Geometry: final body of the model. Coordinates: model frame, mm. Face numbers are marked on the shaded views. A direction names the side the tool comes from. Round coordinates to 2 decimals unless told otherwise and drop trailing zeros. Loops run counter-clockwise (first coordinate to the right, second up) from the corner with the lowest first, then second, coordinate; pieces in that order, holes last. Notation, with made-up numbers: (32, -9) - (86, -9) arc R15 ccw to (86, 20) - close; hole circle Ø7 at (48, 8). An arc over 180 degrees is marked (long way). Answer as CSV lines item,"result".
from build123d import *

# Parameters (mm, degrees)
SWEEP_THIN2_PROFILE_R   = 3.5
SWEEP_THIN2_PROFILE_R_2 = 2.5
SKETCH57_R              = 3.5
SKETCH57_R_2            = 3
BOSS_EXTRUDE1_DEPTH     = 17.5


with BuildPart() as part:
    # Sweep-Thin2: sweep along a path in Sketch28
    with BuildLine(Plane.XY) as sweep_thin2_path:
        Line((-46, -41), (-46, -13))
        ThreePointArc((-46, -13), (-42.192388155, -3.807611845), (-33, 0))
        Line((-33, 0), (33, 0))
        ThreePointArc((33, 0), (42.192388155, -3.807611845), (46, -13))
        Line((46, -13), (46, -41))
    # Sweep-Thin2 profile (on start of the path) → Sweep-Thin2 (sweep)
    with BuildSketch(Plane(origin=(-46, -41, 0), x_dir=(1, 0, 0), z_dir=(0, 1, 0))):
        Circle(SWEEP_THIN2_PROFILE_R)
        Circle(SWEEP_THIN2_PROFILE_R_2, mode=Mode.SUBTRACT)
    sweep(path=sweep_thin2_path.line)

    # Sketch57 → Boss-Extrude1 (add)
    with BuildSketch(Plane.XY):
        with Locations(Location((0, 0, 0), (0, 0, 270))):
            Circle(SKETCH57_R)
        with Locations(Location((0, 0, 0), (0, 0, 180))):
            Circle(SKETCH57_R_2, mode=Mode.SUBTRACT)
    extrude(amount=BOSS_EXTRUDE1_DEPTH)


solid = part.part
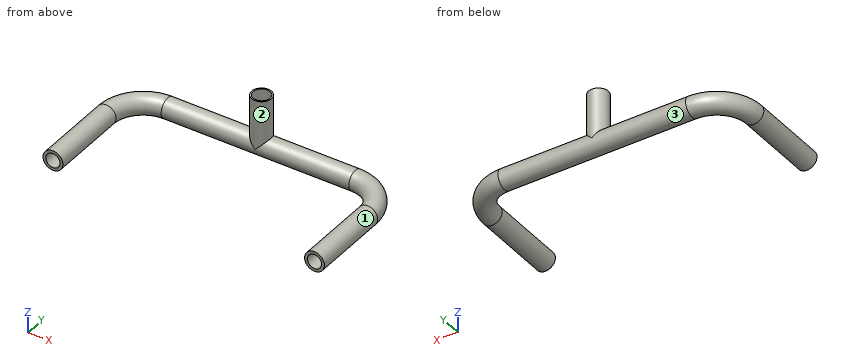
(1) Section A-A (x = 0). Output: boundary loops of the cut face in (y, z), and give its area (3 significant figures).
Findings below:
outline,"(-3.5, 0) arc R3.5 ccw to (3.5, 0) - (3.5, 17.5) - (3, 17.5) - (3, 1.8) arc R3.5 ccw to (-3, 1.8) - (-3, 17.5) - (-3.5, 17.5) - close; hole circle Ø5 at (0, 0)"
area,"35.1 mm2"
(2) Access query for the marked faces 1, 2 and 3. Directions: +Z, -Z, +X, -X, +Y, -Y. A direction counts if a zero-diameter tool reaches every point of the face in a straight line with its end or side. Return the directions, or none.
Findings below:
face 1,"-Y"
face 2,"+Z"
face 3,"none"
(3) Pin query (flat end, axial travel): P1, Ø4.5, axis at x = -46, z = 0, coming from the +Y side; P2, Ø0.9, axis at x = 3, y = 1, coming from the -Z side; P3, Ø1.5, axis at y = -29.5, z = 5, coming from the -X side (3 decimals); P4, Ø8, axis at x = -15, y = -3, coming from the +Z side. Return the tip coordinate at first contact, or that it passes through.
Findings below:
P1,"y = -0.48"
P2,"z = -3.46"
P3,"through"
P4,"z = 3.5"
(4) Section C-C (z = 10). Output: boundary loops of the cut face in (x, y).
Findings below:
outline,"circle Ø7 at (0, 0); hole circle Ø6 at (0, 0)"
(5) Section B-B (y = -33.5). Output: boundary loops of the cut face in (x, z), and give its area (3 significant figures).
Findings below:
outline,"circle Ø7 at (-46, 0); circle Ø7 at (46, 0); hole circle Ø5 at (-46, 0); hole circle Ø5 at (46, 0)"
area,"37.7 mm2"
(6) Material intervals for line 1 along X through (y, z) = (-18.75, 0); line 2 along Z through (x, y) = (-46, -26.25), sorted ascending.
Findings below:
line 1,"-49.5 to -48.5, -43.5 to -42.5, 42.5 to 43.5, 48.5 to 49.5"
line 2,"-3.5 to -2.5, 2.5 to 3.5"
(7) Section D-D (y = -11). Give the number of separate pieces and of enclosed holes in the cut face, and give its area (3 significant figures).
Findings below:
separate pieces,"2"
enclosed holes,"2"
area,"38.2 mm2"
